Geometry: final body of the model. Coordinates: model frame, mm. Face numbers are marked on the shaded views. A direction names the side the tool comes from. Round coordinates to 2 decimals unless told otherwise and drop trailing zeros. Loops run counter-clockwise (first coordinate to the right, second up) from the corner with the lowest first, then second, coordinate; pieces in that order, holes last. Notation, with made-up numbers: (25.5, 5.5) - (77.5, 5.5) arc R18 ccw to (77.5, 15.5) - close; hole circle Ø7 at (54.25, -15). An arc over 180 degrees is marked (long way). Use CSV: the item, a comma, the result in double quotes.
from build123d import *

# Parameters (mm, degrees)
BASE_FEATURE_DEPTH         = 25.4
SKETCH2_W                  = 38.1
SKETCH2_H                  = 19.05
ALTITUDUAL_CUT_DEPTH       = 67.067470248
F_1_2_0_5_DIAMETER_HOLES_D = 12.7


with BuildPart() as part:
    # Sketch1 → Base Feature (new, symmetric)
    with BuildSketch(Plane.XY):
        Polygon((-47.625, 0), (41.275, 0), (41.275, 38.1), (28.575, 38.1), (28.575, 19.05), (-28.575, 19.05), (-28.575, 38.1), (-47.625, 38.1), align=None)
    extrude(amount=BASE_FEATURE_DEPTH, both=True)

    # Sketch2 → Altitudual Cut (cut, through all)
    with BuildSketch(Plane.XZ):
        with Locations((22.225, 15.875)):
            Rectangle(SKETCH2_W, SKETCH2_H)
    extrude(amount=-ALTITUDUAL_CUT_DEPTH, mode=Mode.SUBTRACT)

    # 1/2 (0.5) Diameter Holes (through all)
    with Locations(Plane(origin=(0, 19.05, 0), x_dir=(1, 0, 0), z_dir=(0, 1, 0))):
        with Locations((-15.875, -12.7), (3.175, 12.7)):
            Hole(F_1_2_0_5_DIAMETER_HOLES_D / 2)


solid = part.part
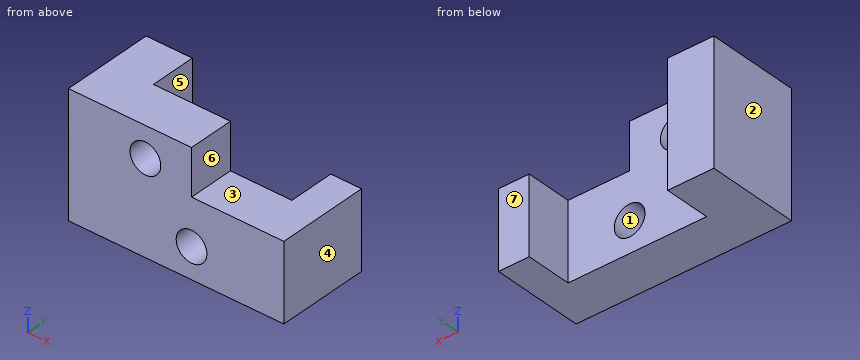
Item 1: Section C-C on z = -12.7. Return the cut outline in (x, y) (3 decimals).
Final values:
outline,"(-47.625, 0) - (-3.175, 0) - (-3.175, 19.05) - (-28.575, 19.05) - (-28.575, 38.1) - (-47.625, 38.1) - close; (9.525, 0) - (41.275, 0) - (41.275, 38.1) - (28.575, 38.1) - (28.575, 19.05) - (9.525, 19.05) - close"
Item 2: Section A-A on z = 12.7. Return the cut outline in (x, y) (3 decimals).
Final values:
outline,"(-47.625, 0) - (-22.225, 0) - (-22.225, 19.05) - (-28.575, 19.05) - (-28.575, 38.1) - (-47.625, 38.1) - close; (-9.525, 0) - (3.175, 0) - (3.175, 19.05) - (-9.525, 19.05) - close"
Item 3: Section D-D on x = 5.5. Return the cut outline in (y, z), plus the area to 3 significant figures.
Final values:
outline,"(0, -25.4) - (19.05, -25.4) - (19.05, -18.61) - (0, -18.61) - close; (0, -6.79) - (19.05, -6.79) - (19.05, 6.35) - (0, 6.35) - close"
area,"380 mm²"
Item 4: Section B-B on y = 31. Return the cut outline in (x, z) (3 decimals).
Final values:
outline,"(-47.625, -25.4) - (-28.575, -25.4) - (-28.575, 25.4) - (-47.625, 25.4) - close; (28.575, -25.4) - (41.275, -25.4) - (41.275, 6.35) - (28.575, 6.35) - close"
Item 5: Reachability of the marked faces 5, 6 and 7 from +Z, -Z, +X, -X, +Y, -Y: full face, straight path, thin tool, end or side. Return the list, or none.
Final values:
face 5,"+Z, -Z, +Y"
face 6,"+Z, +X, +Y, -Y"
face 7,"+Z, -Z, +X, -X, +Y"
Item 6: Pin query (flat end, axial travel): P1, Ø12, axis at x = -14, z = 15.5, coming from the -Y side; P2, Ø12, axis at x = 8.5, z = -9, coming from the +Y side; P3, Ø19, axis at x = 31.5, y = 10, coming from the +Z side. Return the tip coordinate at first contact, or that it passes through.
Final values:
P1,"stops at y = 0"
P2,"stops at y = 19.05"
P3,"stops at z = 6.35"
Item 7: Mould query, pull axis X, two halves, no side actions, for the marked faces 1, 2, 3 and 4. Classes: released by +X, released by -X, zero draft, split by the parting line, or undercut.
Final values:
face 1,"undercut"
face 2,"released by -X"
face 3,"zero draft"
face 4,"released by +X"
Item 8: Material intervals for line 1 (X direction, y = 25.5, z = -8.5) (3 decimals); line 2 (X direction, y = 21, z = 21) (3 decimals); line 3 (X direction, y = 7, z = 22) (3 decimals), sorted ascending.
Final values:
line 1,"x = -47.625 to -28.575, 28.575 to 41.275"
line 2,"x = -47.625 to -28.575"
line 3,"x = -47.625 to 3.175"
